For this review, take the finished solid that the model builds, in its own axes (mm). Face numbers are marked on the shaded views. Round coordinates to 2 decimals unless told otherwise and drop trailing zeros. Loops run counter-clockwise (first coordinate to the right, second up) from the corner with the lowest first, then second, coordinate; pieces in that order, holes last. Notation, with made-up numbers: M 53.5,18.5 L 71.5,18.5 A17 ccw 71.5,38.5 Z; hole C -15,13 d4. An arc over 180 degrees is marked long. One line per question, with ' | ' between items. Start each with the question number.
1) We need section B-B (y = -26.5). Give the boundary of the cut face in (x, z).
2) We need section C-C (x = 64). Give the boundary of the cut face in (y, z), and give its area (3 significant figures).
3) For pin 1 Ø4 at (y, z) = (-196.5, 125.5) entering from +X; pin 2 Ø2 at (y, z) = (-162.5, 118.5) entering from +X; pin 3 Ø3 at (y, z) = (-209.5, 143.5) entering from +X, all flat-tipped, find the tip position at first contact; note any pin that passes through.
4) We need section D-D (z = 139.5). Give the boundary of the cut face in (x, y).
5) Mouldability with a two-part tool opening along Z and no side actions: class the marked faces 1, 2 and 3 as pulls with the +Z half, pulls with the -Z half, needs draft (parallel to the pull), parting line crosses it, or undercut.
6) We need section A-A (x = 193). Give the boundary of the cut face in (y, z), and give its area (3 significant figures).
7) For probe 1 along Z at (x, y) = (168, -109.5); probe 2 along Z at (x, y) = (236.5, -144); probe 3 along Z at (x, y) = (281, -101), list the stretches that pass through material, from the lowest coordinate up. Write a range as from..to.
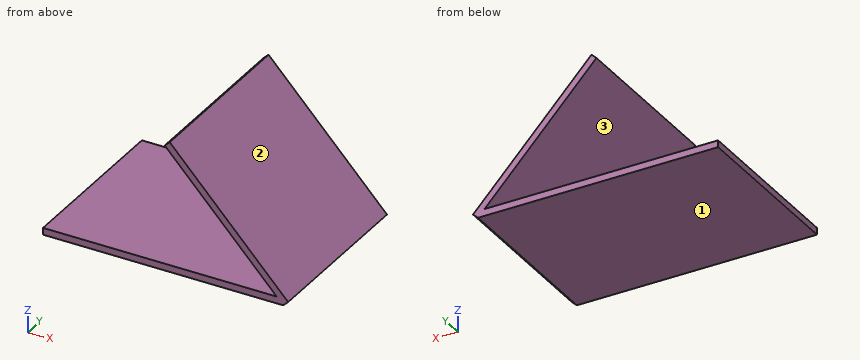
Autodesk Inventor part; units mm, degrees
ref_plane "Plano de trabajo1" through (350, -250, 0) normal (-0.7285, 0, -0.685) x (0, 1, 0)
ref_plane "YZ Plane" through (0, 0, 0) normal (1, 0, 0) x (0, 1, 0)
ref_plane "XZ Plane" through (0, 0, 0) normal (0, 1, 0) x (-1, 0, 0)
sketch "Boceto1" plane through (0, 0, 0) normal (0, 0, 1) x (1, 0, 0)
  line L0 (0, 0) -> (350, 0)
  line L1 (350, 0) -> (350, -250)
  line L2 (350, -250) -> (0, -250)
  line L3 (0, -250) -> (0, 0)
  dimension "d0" = 350
  dimension "d1" = 250
extrude "Extrusión1" add sketch "Boceto1" along normal blind 10
ref_plane "Plano de trabajo1" through (350, -250, 0) normal (-0.7285, 0, -0.685) x (0, 1, 0)
sketch "Boceto2" plane through (350, -250, 0) normal (-0.7285, 0, -0.685) x (0, 1, 0)
  line L0 (0, 0) -> (250, 0)
  line L1 (0, 0) -> (250, 0)
  line L2 (250, 0) -> (250, -252)
  line L3 (250, -252) -> (0, -252)
  line L4 (0, -252) -> (0, 0)
  point P0 (250, -239.7606)
  point P1 (250, 0)
  dimension "d5" = 250
  dimension "d6" = 252
extrude "Extrusión2" add sketch "Boceto2" against normal blind 10
sketch "Boceto3" plane through (357.2851, -250, 6.8503) normal (0.7285, 0, 0.685) x (0.685, 0, -0.7285)
  arc A0 (-179.2335, 22.3949) -> (-179.2335, 102.4229) centre (-179.2335, 62.4089) ccw
  line L0 (-179.2335, 22.3949) -> (-205.9095, 22.3949)
  line L1 (-205.9095, 22.3949) -> (-205.9095, 89.0849)
  line L2 (-179.2335, 89.0849) -> (-192.5715, 89.0849)
  line L3 (-192.5715, 89.0849) -> (-192.5715, 35.7329)
  line L4 (-192.5715, 35.7329) -> (-179.2335, 35.7329)
  arc A1 (-179.2335, 35.7329) -> (-179.2335, 89.0849) centre (-179.2335, 62.4089) ccw
  line L5 (-192.5715, 89.0849) -> (-205.9095, 89.0849)
  line L6 (-192.5715, 102.4229) -> (-192.5715, 89.0849)
  line L7 (-200.5743, 127.8046) -> (-200.5743, 117.1342)
  line L8 (-200.5743, 117.1342) -> (-157.8927, 117.1342)
  line L9 (-157.8927, 117.1342) -> (-157.8927, 127.8046)
  arc A2 (-157.8927, 127.8046) -> (-200.5743, 127.8046) centre (-179.2335, 127.8046) ccw
  line L10 (-200.5743, 160.5789) -> (-203.2419, 160.5789)
  line L11 (-200.5743, 160.5789) -> (-197.9067, 160.5789)
  line L12 (-191.2377, 160.5789) -> (-157.8927, 160.5789)
  line L13 (-200.5743, 183.5325) -> (-200.5743, 172.8621)
  line L14 (-200.5743, 172.8621) -> (-157.8927, 172.8621)
  arc A3 (-157.8927, 183.5325) -> (-200.5743, 183.5325) centre (-179.2335, 183.5325) ccw
  line L15 (-157.8927, 172.8621) -> (-157.8927, 183.5325)
  line L16 (-200.5743, 216.4887) -> (-203.2419, 216.4887)
  line L17 (-200.5743, 216.4887) -> (-197.9067, 216.4887)
  line L18 (-191.2377, 216.4887) -> (-157.8927, 216.4887)
  line L19 (-192.5715, 102.4229) -> (-179.2335, 102.4229)
  line L20 (-75.4492, 148.487) -> (-58.3492, 148.487)
  line L21 (-58.3492, 170.7597) -> (-64.3342, 170.7597)
  line L22 (-92.5492, 135.662) -> (-75.4492, 148.487)
  line L23 (-92.5492, 161.312) -> (-75.4492, 148.487)
  line L24 (-92.5492, 180.5891) -> (-58.3492, 193.4141)
  line L25 (-92.5492, 206.2391) -> (-58.3492, 193.4141)
  line L26 (-58.3492, 215.852) -> (-64.3342, 215.852)
  line L27 (-58.6269, 85.751) -> (-92.8269, 85.751)
  arc A4 (-71.4519, 98.576) -> (-92.8269, 98.576) centre (-82.1394, 98.576) ccw
  line L28 (-71.4519, 98.576) -> (-71.4519, 85.751)
  line L29 (-58.6269, 30.982) -> (-92.8269, 39.532)
  line L30 (-92.8269, 39.532) -> (-58.6269, 48.082)
  line L31 (-92.8269, 56.632) -> (-58.6269, 48.082)
  line L32 (-92.8269, 56.632) -> (-58.6269, 65.182)
  line L33 (-58.6269, 75.322) -> (-64.6119, 75.322)
  line L34 (-92.8269, 85.751) -> (-92.8269, 98.576)
  line L35 (-58.6269, 118.6704) -> (-64.6119, 118.6704)
  point P0 (-239.7606, 250)
  point P1 (-58.6269, 30.982)
properties part number "Logo_names"
Answers below:
1) outline: M 0,0 L 350,0 L 357.29,6.85 L 184.66,190.44 L 177.37,183.59 L 340.6,10 L 0,10 Z
2) outline: M -250,0 L 0,0 L 0,10 L -250,10 Z | area: 2,500 mm^2
3) pin 1: x = 247.6 | pin 2: x = 253.24 | pin 3: x = 230.21
4) outline: M 218.83,-250 L 232.56,-250 L 232.56,0 L 218.83,0 Z
5) face 1: pulls with the -Z half | face 2: pulls with the +Z half | face 3: undercut
6) outline: M -250,0 L 0,0 L 0,10 L -250,10 Z; M -250,166.97 L 0,166.97 L 0,181.57 L -250,181.57 Z | area: 6,150 mm^2
7) probe 1: 0..10 | probe 2: 0..10, 120.71..135.31 | probe 3: 0..10, 73.38..87.98
